Can you work these out from the model? Positions are in its coordinate system, mm. A direction names the side the tool comes from. Give positions to 0.01 mm unless a question says otherwise; leave off trailing zeros. Order: outer loops, then holes, each group sorted by start corner. A loop starts at its lowest first (then second) coordinate and runs counter-clockwise, first axis right, second up. Notation, with made-up numbers: (12, 1) - (35, 1) arc R17 ccw to (35, 30) - close; hole circle Ø8 at (43.5, 29). An arc over 180 degrees is marked (long way). Answer as a JSON object with one key per item and string values.
```python
from build123d import *

# Parameters (mm, degrees)
PAD_DEPTH       = 10
SKETCH001_R     = 3.4
POCKET_DEPTH    = 10.001
PAD001_DEPTH    = 5
POCKET001_DEPTH = 5
SKETCH004_W     = 3.2
SKETCH004_H     = 10
POCKET002_DEPTH = 3
SKETCH005_W     = 3.2
SKETCH005_H     = 7
POCKET003_DEPTH = 3
SKETCH006_W     = 3.2
SKETCH006_H     = 7
POCKET004_DEPTH = 3


with BuildPart() as part:
    # Sketch → Pad (new body)
    with BuildSketch(Plane.XZ):
        Polygon((0.868689, 3.613865), (-52.131311, 3.613865), (-52.131311, 5.613865), (-54.131311, 5.613865), (-54.131311, 3.613865), (-62.131311, 3.613865), (-62.131311, 13.613865), (-38.323146, 13.613865), (0.868689, 5.613865), align=None)
    extrude(amount=PAD_DEPTH)

    # Sketch001 → Pocket (cut, through all)
    with BuildSketch(Plane.XZ.offset(10)):
        with Locations((-34.923146, 13.613865)):
            Circle(SKETCH001_R)
    extrude(amount=-POCKET_DEPTH, mode=Mode.SUBTRACT)

    # Sketch002 → Pad001 (new body)
    with BuildSketch(Plane.XZ.offset(10)):
        Polygon((-48.323146, 13.613865), (-48.323146, 17.613865), (-50.323146, 17.613865), (-54.323146, 13.613865), align=None)
    extrude(amount=-PAD001_DEPTH)

    # Sketch003 → Pocket001 (cut)
    with BuildSketch(Plane(origin=(0, 0, 0), x_dir=(1, 0, 0), z_dir=(0, 1, 0))):
        Polygon((-48.323146, -13.613865), (-48.323146, -9.613865), (-50.323146, -9.613865), (-54.323146, -13.613865), align=None)
    extrude(amount=-POCKET001_DEPTH, mode=Mode.SUBTRACT)

    # Sketch004 → Pocket002 (cut)
    with BuildSketch(Plane(origin=(0, 0, 13.613865), x_dir=(-1, 0, 0), z_dir=(0, 0, 1))):
        with Locations((58.531311, 5)):
            Rectangle(SKETCH004_W, SKETCH004_H)
    extrude(amount=-POCKET002_DEPTH, mode=Mode.SUBTRACT)

    # Sketch005 → Pocket003 (cut)
    with BuildSketch(Plane.XZ.offset(10)):
        with Locations((-58.531311, 7.113865)):
            Rectangle(SKETCH005_W, SKETCH005_H)
    extrude(amount=-POCKET003_DEPTH, mode=Mode.SUBTRACT)

    # Sketch006 → Pocket004 (cut)
    with BuildSketch(Plane(origin=(0, 0, 0), x_dir=(1, 0, 0), z_dir=(0, 1, 0))):
        with Locations((-58.531311, -7.113865)):
            Rectangle(SKETCH006_W, SKETCH006_H)
    extrude(amount=-POCKET004_DEPTH, mode=Mode.SUBTRACT)


solid = part.part
```
Q1. I need wall thicknesses on L1, parallel to X at y = -1.75, z = 5.5; L2, parallel to Y at x = -50.5, z = 11.5; L3, parallel to Z at x = -35, y = -8.5. Which ranges of each line are inside material? Lowest first, please.
Recorded:
{"L1": "x = -62.13 to -60.13, -56.93 to -54.13, -52.13 to 0.87", "L2": "y = -10 to -5", "L3": "z = 3.61 to 10.21"}
Q2. If we section it at A-A, the plane y = -1: Please give me the cut outline in (x, z), then the cut area to 3 significant figures.
Recorded:
{"outline": "(-62.13, 3.61) - (-60.13, 3.61) - (-60.13, 13.61) - (-62.13, 13.61) - close; (-56.93, 3.61) - (-54.13, 3.61) - (-54.13, 5.61) - (-52.13, 5.61) - (-52.13, 3.61) - (0.87, 3.61) - (0.87, 5.61) - (-31.8, 12.28) arc R3.4 cw to (-38.32, 13.61) - (-48.32, 13.61) - (-48.32, 9.61) - (-50.32, 9.61) - (-54.32, 13.61) - (-56.93, 13.61) - close", "area": "408 mm^2"}
Q3. Which directions (+Z, -Z, +X, -X, +Y, -Y) give clear straight access to the entire face, cutting with the end or side of a thin tool? Please do faces 1 (the face through (-59, -7, 7)), 2 (the face through (-60.131, -5, 11)), 3 (the face through (-59, -5, 10.614)).
Recorded:
{"face 1": "+Z, -Z, -Y", "face 2": "+Z", "face 3": "+Z, +Y, -Y"}
Q4. If we section it at D-D, the plane y = -8.5: Please give me the cut outline in (x, z).
Recorded:
{"outline": "(-62.13, 3.61) - (-60.13, 3.61) - (-60.13, 13.61) - (-62.13, 13.61) - close; (-56.93, 3.61) - (-54.13, 3.61) - (-54.13, 5.61) - (-52.13, 5.61) - (-52.13, 3.61) - (0.87, 3.61) - (0.87, 5.61) - (-31.8, 12.28) arc R3.4 cw to (-38.32, 13.61) - (-48.32, 13.61) - (-48.32, 17.61) - (-50.32, 17.61) - (-54.32, 13.61) - (-56.93, 13.61) - close"}
Q5. If we section it at B-B, the plane z = 13: Please give me the cut outline in (x, y).
Recorded:
{"outline": "(-62.13, -10) - (-60.13, -10) - (-60.13, 0) - (-62.13, 0) - close; (-56.93, -10) - (-38.27, -10) - (-38.27, 0) - (-48.32, 0) - (-48.32, -5) - (-53.71, -5) - (-53.71, 0) - (-56.93, 0) - close"}
Q6. We'd pull the mould along X, two halves only. Please class faces 4 (the face through (-58, -5, 3.614)), 5 (the face through (0.869, -5, 5)), 6 (the face through (-54.131, -5, 5)): released by +X, released by -X, zero draft, split by the parting line, or undercut.
Recorded:
{"face 4": "zero draft", "face 5": "released by +X", "face 6": "undercut"}
Q7. If we section it at C-C, the plane y = -4: Please give me the cut outline in (x, z).
Recorded:
{"outline": "(-62.13, 3.61) - (-54.13, 3.61) - (-54.13, 5.61) - (-52.13, 5.61) - (-52.13, 3.61) - (0.87, 3.61) - (0.87, 5.61) - (-31.8, 12.28) arc R3.4 cw to (-38.32, 13.61) - (-48.32, 13.61) - (-48.32, 9.61) - (-50.32, 9.61) - (-54.32, 13.61) - (-56.93, 13.61) - (-56.93, 10.61) - (-60.13, 10.61) - (-60.13, 13.61) - (-62.13, 13.61) - close"}
Q8. I'm going to push flat-ended pins straight in: pin 1 Ø0.6 at (x, y) = (-53, -7) entering from -Z; pin 2 Ø1.6 at (x, y) = (-61, -6.5) entering from +Z; pin 3 Ø5 at (x, y) = (-5.5, -4.5) entering from +Z. Where does each tip first touch, or does it pass through?
Recorded:
{"pin 1": "stops at z = 5.61", "pin 2": "stops at z = 13.61", "pin 3": "stops at z = 7.42"}
